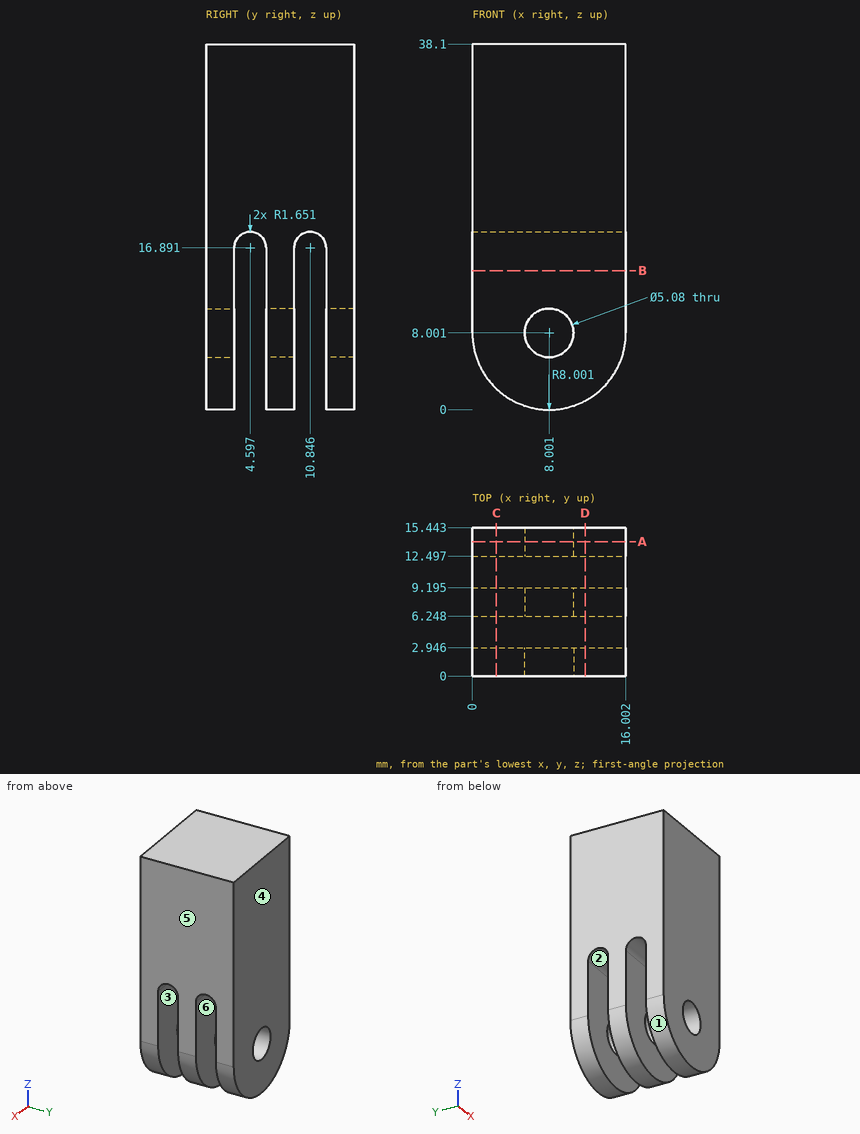
Design review of the part shown in the three views and the two pictorial views. Dimensions are in mm from the part's minimum x, y and z. A direction names the side the tool comes from. Round coordinates to 2 decimals unless told otherwise and drop trailing zeros. Order: outer loops, then holes, each group sorted by start corner. A loop starts at its lowest first (then second) coordinate and runs counter-clockwise, first axis right, second up.
Item 1: For pin 1 (2 mm diameter, centred on y = 6.5, z = 9, fed in from -X); pin 2 (1 mm diameter, centred on y = 11, z = 7, fed in from -X) (3 decimals), all flat-tipped, find the tip position at first contact; note any pin that passes through.
Working result:
pin 1: stops at x = 0
pin 2: passes through
Item 2: To check wall thickness, follow probe 1 along Y at (x, z) = (6, 15) (1 decimal); probe 2 along Y at (x, z) = (4.25, 18) (1 decimal); probe 3 along Z at (x, y) = (7, 1) (1 decimal). State the ranges of each line that lie inside material, in increasing order.
Working result:
probe 1: y = 0 to 2.9, 6.2 to 9.2, 12.5 to 15.4
probe 2: y = 0 to 3.4, 5.8 to 9.6, 12.1 to 15.4
probe 3: z = 0.1 to 5.7, 10.3 to 38.1
Item 3: Draft analysis for pull direction Y (two halves, no side actions). For the marked faces 1, 2, 3 and 4, state which applies: released by +Y, released by -Y, zero draft, split by the parting line, or undercut.
Working result:
face 1: zero draft
face 2: undercut
face 3: undercut
face 4: released by +Y
Item 4: Add section B-B, the plane z = 14.5. State the section outline as (x, y) points (1 decimal).
Working result:
outline: (0, 0) - (16, 0) - (16, 2.9) - (0, 2.9) - close; (0, 6.2) - (16, 6.2) - (16, 9.2) - (0, 9.2) - close; (0, 12.5) - (16, 12.5) - (16, 15.4) - (0, 15.4) - close
Item 5: Add section A-A, the plane y = 14. State the section outline as (x, z) points.
Working result:
outline: (0, 8) arc R8 ccw to (16, 8) - (16, 38.1) - (0, 38.1) - close; hole circle Ø5.08 at (8, 8)
Item 6: Add section C-C, the plane x = 2.5. State the section outline as (y, z) points (1 decimal), and give its area (3 significant figures).
Working result:
outline: (0, 2.2) - (2.9, 2.2) - (2.9, 16.9) arc R1.7 cw to (6.2, 16.9) - (6.2, 2.2) - (9.2, 2.2) - (9.2, 16.9) arc R1.7 cw to (12.5, 16.9) - (12.5, 2.2) - (15.4, 2.2) - (15.4, 38.1) - (0, 38.1) - close
area: 449 mm2
Item 7: Machinability: for the marked faces 5 and 6, which of the approach directions +Z, -Z, +X, -X, +Y, -Y give a long, thin tool a straight path to every point of the face, cutting with its end or side? Answer none if there is none.
Working result:
face 5: +Z, -Z, +X, +Y, -Y
face 6: -Z, +X, -X
Item 8: Add section D-D, the plane x = 11.75. State the section outline as (y, z) points (1 decimal).
Working result:
outline: (0, 0.9) - (2.9, 0.9) - (2.9, 16.9) arc R1.7 cw to (6.2, 16.9) - (6.2, 0.9) - (9.2, 0.9) - (9.2, 16.9) arc R1.7 cw to (12.5, 16.9) - (12.5, 0.9) - (15.4, 0.9) - (15.4, 38.1) - (0, 38.1) - close
